Can you work these out from the model? Positions are in its coordinate system, mm. Face numbers are marked on the shaded views. Round coordinates to 2 decimals unless told otherwise and drop trailing zeros. Loops run counter-clockwise (first coordinate to the right, second up) from the corner with the lowest first, then second, coordinate; pieces in that order, holes last.
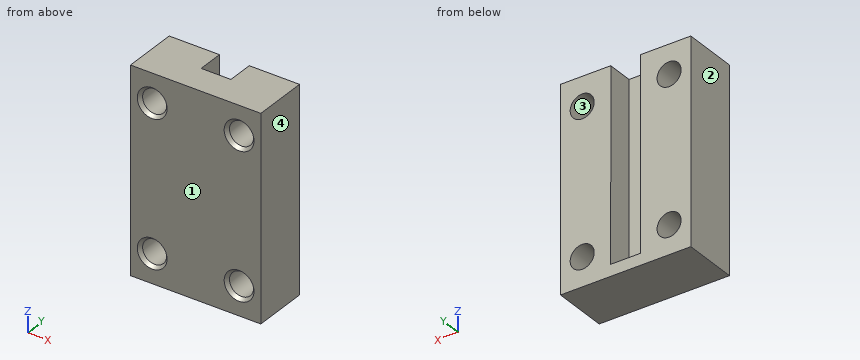
from build123d import *

# Parameters (mm, degrees)
SKETCH1_W           = 45
SKETCH1_H           = 70
BOSS_EXTRUDE1_DEPTH = 10
SKETCH3_R           = 4.15
CUT_EXTRUDE2_DEPTH  = 11
SKETCH5_R           = 4.15
BOSS_EXTRUDE2_DEPTH = 9
CHAMFER1_SIZE       = 1
CHAMFER1_SIZE2      = 1.191753593


with BuildPart() as part:
    # Sketch1 → Boss-Extrude1 (new body)
    with BuildSketch(Plane(origin=(0, 0, 0), x_dir=(1, 0, 0), z_dir=(0, 1, 0))):
        Rectangle(SKETCH1_W, SKETCH1_H)
    extrude(amount=BOSS_EXTRUDE1_DEPTH)

    # Sketch3 → Cut-Extrude2 (cut, through all)
    with BuildSketch(Plane.XZ):
        with Locations((15, 25)):
            Circle(SKETCH3_R)
        with Locations((15, -25)):
            Circle(SKETCH3_R)
        with Locations((-15, -25)):
            Circle(SKETCH3_R)
        with Locations((-15, 25)):
            Circle(SKETCH3_R)
    extrude(amount=-CUT_EXTRUDE2_DEPTH, mode=Mode.SUBTRACT)

    # Sketch5 → Boss-Extrude2 (add)
    with BuildSketch(Plane(origin=(0, 10, 0), x_dir=(1, 0, 0), z_dir=(0, 1, 0))):
        Polygon((-5.15, -35), (-22.5, -35), (-22.5, 35), (22.5, 35), (22.5, -35), (5.15, -35), (5.130229348, -34.949305848), (5.15, 31), (-5.15, 31), align=None)
        with Locations((-15, 25)):
            Circle(SKETCH5_R, mode=Mode.SUBTRACT)
        with Locations((15, 25)):
            Circle(SKETCH5_R, mode=Mode.SUBTRACT)
        with Locations((15, -25)):
            Circle(SKETCH5_R, mode=Mode.SUBTRACT)
        with Locations((-15, -25)):
            Circle(SKETCH5_R, mode=Mode.SUBTRACT)
    extrude(amount=BOSS_EXTRUDE2_DEPTH)

    # Chamfer1
    chamfer1_edges = [part.edges().sort_by_distance(p)[0] for p in [
        (-19.15, 0, -25),
        (-19.15, 0, 25),
        (10.85, 0, 25),
        (10.85, 0, -25),
    ]]
    chamfer1_side = [part.faces().sort_by_distance(p)[0] for p in [
        (0, 0, 0),
    ]]
    chamfer(chamfer1_edges, length=CHAMFER1_SIZE, length2=CHAMFER1_SIZE2, reference=chamfer1_side[0])


solid = part.part
(1) If we mould it in two halves opening along X, with no side actions, what happens to the marked faces 1, 2, 3 and 4? For each: released by +X, released by -X, zero draft, split by the parting line, or undercut.
Worked answers:
face 1: zero draft
face 2: released by -X
face 3: undercut
face 4: released by +X
(2) If we section it at B-B, the plane y = 15.25: List the corners of the cut face in (x, z) for me.
Worked answers:
outline: (-22.5, -35) - (22.5, -35) - (22.5, 35) - (5.15, 35) - (5.13, 34.95) - (5.15, -31) - (-5.15, -31) - (-5.15, 35) - (-22.5, 35) - close; hole circle Ø8.3 at (-15, -25); hole circle Ø8.3 at (-15, 25); hole circle Ø8.3 at (15, -25); hole circle Ø8.3 at (15, 25)
(3) If I drill on line 1 (X direction, y = 14.75, z = 25); line 2 (Z direction, x = 15, y = 10.25); line 3 (X direction, y = 8.5, z = -25), over which ranges is the centre line in solid material (lowest first)?
Worked answers:
line 1: x = -22.5 to -19.15, -10.85 to -5.15, 5.13 to 10.85, 19.15 to 22.5
line 2: z = -35 to -29.15, -20.85 to 20.85, 29.15 to 35
line 3: x = -22.5 to -19.15, -10.85 to 10.85, 19.15 to 22.5
(4) If we section it at D-D, the plane x = -4: List the corners of the cut face in (y, z) for me, then the cut area to 3 significant figures.
Worked answers:
outline: (0, -35) - (19, -35) - (19, -31) - (10, -31) - (10, 35) - (0, 35) - close
area: 736 mm2
(5) If we section it at C-C, the plane z = 25: List the corners of the cut face in (x, y) for me, then the cut area to 3 significant figures.
Worked answers:
outline: (-22.5, 0) - (-20.15, 0) - (-19.15, 1.19) - (-19.15, 19) - (-22.5, 19) - close; (-10.85, 1.19) - (-9.85, 0) - (9.85, 0) - (10.85, 1.19) - (10.85, 19) - (5.13, 19) - (5.13, 10) - (-5.15, 10) - (-5.15, 19) - (-10.85, 19) - close; (19.15, 1.19) - (20.15, 0) - (22.5, 0) - (22.5, 19) - (19.15, 19) - close
area: 445 mm2
(6) Will these pins go through, and if not, where does the flat tip stop? P1, Ø5, axis at x = 2, z = 17, coming from the +Y side; P2, Ø2.5, axis at x = 1.5, y = 16.5, coming from the +Z side.
Worked answers:
P1: stops at y = 10
P2: stops at z = -31
(7) If we section it at A-A, the plane x = -15: List the corners of the cut face in (y, z) for me.
Worked answers:
outline: (0, -35) - (19, -35) - (19, -29.15) - (1.19, -29.15) - (0, -30.15) - close; (0, -19.85) - (1.19, -20.85) - (19, -20.85) - (19, 20.85) - (1.19, 20.85) - (0, 19.85) - close; (0, 30.15) - (1.19, 29.15) - (19, 29.15) - (19, 35) - (0, 35) - close
